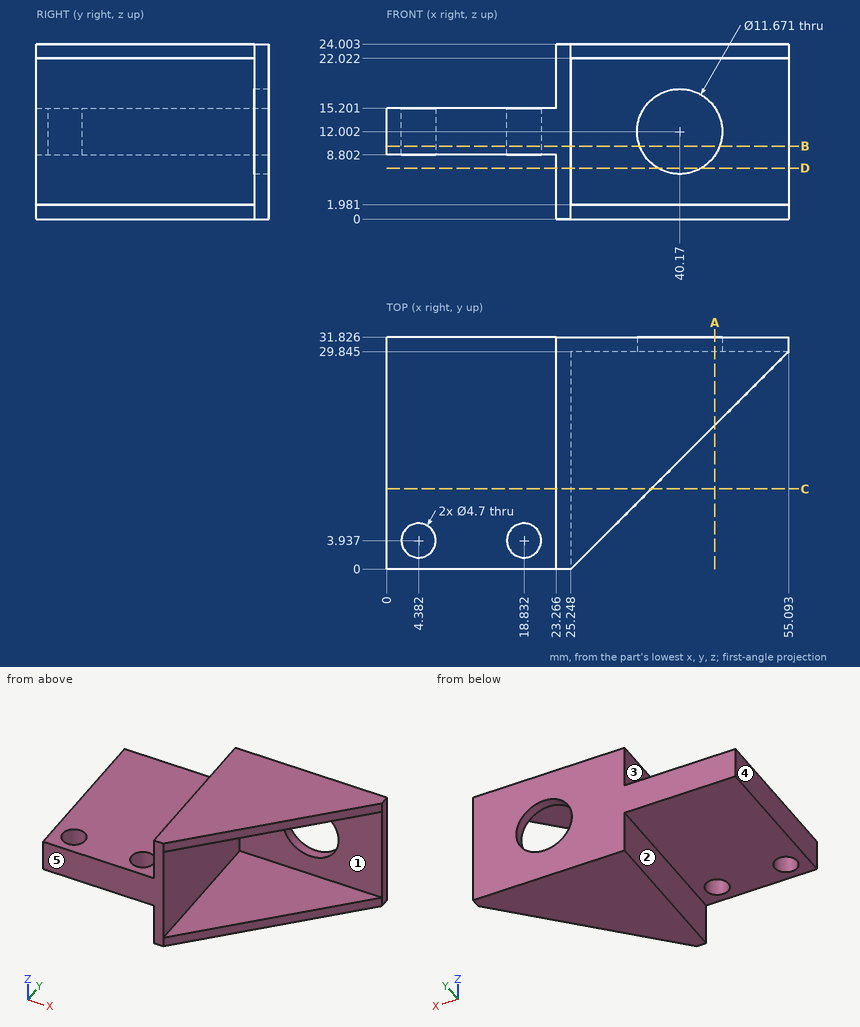
Check sheet for the drawn part. Datum: minimum x, y, z corner. Units: mm. A direction names the side the tool comes from. Coordinates: 2 decimals unless noted, no trailing zeros. Loops run counter-clockwise (first coordinate to the right, second up) from the corner with the lowest first, then second, coordinate; pieces in that order, holes last. Notation, with made-up numbers: (-24.5, -19) -> (26.5, -19) arc R32 ccw to (26.5, 9) -> close; hole circle Ø9 at (-5.5, 65.25). An arc over 180 degrees is marked (long way). Write each question's results on one line, items separated by ' | '.
Item 1: Gauge pin test, flat ends, axial feed: pin 1 (8 mm diameter, centred on x = 18.5, z = 3, fed in from +Y); pin 2 (11.5 mm diameter, centred on x = 11, y = 10.5, fed in from +Z); pin 3 (11.5 mm diameter, centred on x = 14, y = 9.5, fed in from -Z); pin 4 (7 mm diameter, centred on y = 13, z = 19, fed in from -X). Record the tip position at first contact, or that the pin passes through.
Found:
pin 1: passes through | pin 2: stops at z = 15.2 | pin 3: stops at z = 8.8 | pin 4: stops at x = 23.27
Item 2: Section check B-B, the plane z = 10. Count the separate pieces of the cut face and the enclosed holes in it, plus the area to 3 significant figures.
Found:
separate pieces: 2 | enclosed holes: 2 | area: 806 mm2
Item 3: Section check D-D, the plane z = 7. Enter the section's corners in (x, y) (1 decimal).
Found:
outline: (23.3, 0) -> (25.2, 0) -> (25.2, 29.8) -> (37.2, 29.8) -> (37.2, 31.8) -> (23.3, 31.8) -> close; (43.2, 29.8) -> (55.1, 29.8) -> (55.1, 31.8) -> (43.2, 31.8) -> close
Item 4: Section check C-C, the plane y = 11. Enter the section's corners in (x, z), plus the area to 3 significant figures.
Found:
outline: (0, 8.8) -> (23.27, 8.8) -> (23.27, 0) -> (36.25, 0) -> (36.25, 1.98) -> (25.25, 1.98) -> (25.25, 22.02) -> (36.25, 22.02) -> (36.25, 24) -> (23.27, 24) -> (23.27, 15.2) -> (0, 15.2) -> close | area: 240 mm2
Item 5: Material ranges on L1, parallel to Z at x = 27, y = 10.5; L2, parallel to Y at x = 35, z = 2.25 (1 decimal); L3, parallel to X at y = 27, z = 20.5, recorded low to high.
Found:
L1: z = 0 to 1.98, 22.02 to 24 | L2: y = 29.8 to 31.8 | L3: x = 23.27 to 25.25
Item 6: Tool access check on the marked faces 1, 2, 3, 4 and 5. Record the directions out of +Z, -Z, +X, -X, +Y, -Y that give a thin tool (end or side, any length) a straight path to the whole face; none if there is none.
Found:
face 1: +X, -Y | face 2: -Z, -X, +Y, -Y | face 3: +Z, -X, +Y, -Y | face 4: +Z, -Z, -X, +Y, -Y | face 5: +Z, -Z, +X, -X, -Y
Item 7: Section check A-A, the plane x = 45. Enter the section's corners in (y, z) (1 decimal).
Found:
outline: (19.8, 0) -> (31.8, 0) -> (31.8, 8.7) -> (29.8, 8.7) -> (29.8, 2) -> (19.8, 2) -> close; (19.8, 22) -> (29.8, 22) -> (29.8, 15.3) -> (31.8, 15.3) -> (31.8, 24) -> (19.8, 24) -> close
